For this review, take the finished solid that the model builds, in its own axes (mm). Face numbers are marked on the shaded views. Coordinates: 2 decimals unless noted, no trailing zeros. Loops run counter-clockwise (first coordinate to the right, second up) from the corner with the lowest first, then second, coordinate; pieces in that order, holes last. Notation, with made-up numbers: (27.5, 10) - (39.5, 10) arc R15 ccw to (39.5, 34) - close; hole circle Ø3 at (69, 39). An arc over 180 degrees is marked (long way). Answer as a JSON object with one key per item and string values. Group by question number.
Item 1: We need section B-B (x = 0). State how many separate pieces and enclosed holes the cut face has, then the cut area to 3 significant figures.
Item 2: We need section A-A (y = -5.5). Give the boundary of the cut face in (x, z), then the cut area to 3 significant figures.
Item 3: To check wall thickness, follow line 1 (Z direction, x = 0, y = -4.25); line 2 (Z direction, x = -16, y = -7.25); line 3 (X direction, y = -9, z = 7.5). State the ranges of each line that lie inside material, in increasing order.
Item 4: Mouldability with a two-part tool opening along X and no side actions: class the marked faces 1, 2, 3 and 4 as released by +X, released by -X, zero draft, split by the parting line, or undercut.
Item 5: Clearance check with flat-ended pins moving along their axes: pin 1 (3 mm diameter, centred on x = 2, z = 15.5, fed in from -Y); pin 2 (8 mm diameter, centred on x = 15, z = -2, fed in from -Y). State where each tip first meets the part, or that it passes through.
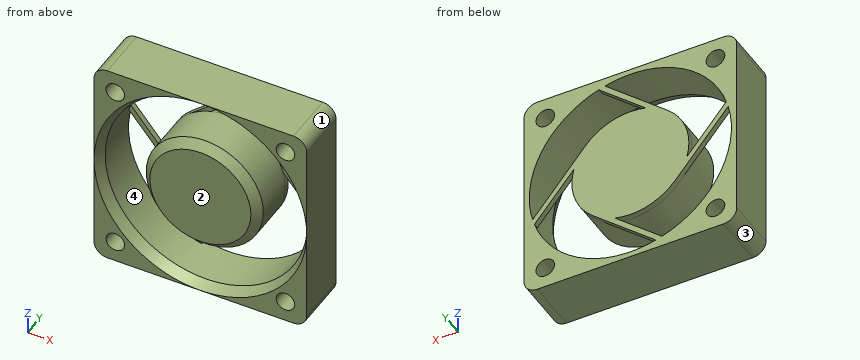
from build123d import *

# Parameters (mm, degrees)
F0_R     = 1.75
F0_R_2   = 19
F1_DEPTH = 10
F3_DEPTH = 1
F4_R     = 11
F5_DEPTH = 9
F7_SIZE2 = 0.99999
F7_SIZE  = 1.99999


# Not quite as in the source:
# - a fillet or chamfer that OpenCascade refuses, or shapes differently, is made with other operations: its cross-section is extruded or revolved along the edge and cut away or added
# - a fillet or chamfer is up to 0.001 mm smaller than in the source, because OpenCascade refuses the exact size


with BuildPart() as f1:
    # F0 (on Front) → F1 (new body)
    with BuildSketch(Plane.XZ):
        with BuildLine():
            Line((-17.5, -20), (17.5, -20))
            ThreePointArc((17.5, -20), (19.267766953, -19.267766953), (20, -17.5))
            Line((20, -17.5), (20, 17.5))
            ThreePointArc((20, 17.5), (19.267766953, 19.267766953), (17.5, 20))
            Line((17.5, 20), (-17.5, 20))
            ThreePointArc((-17.5, 20), (-19.267766953, 19.267766953), (-20, 17.5))
            Line((-20, 17.5), (-20, -17.5))
            ThreePointArc((-20, -17.5), (-19.267766953, -19.267766953), (-17.5, -20))
        make_face()
        with Locations((-16, -16)):
            Circle(F0_R, mode=Mode.SUBTRACT)
        with Locations((16, -16)):
            Circle(F0_R, mode=Mode.SUBTRACT)
        with Locations((-16, 16)):
            Circle(F0_R, mode=Mode.SUBTRACT)
        Circle(F0_R_2, mode=Mode.SUBTRACT)
        with Locations((16, 16)):
            Circle(F0_R, mode=Mode.SUBTRACT)
    extrude(amount=F1_DEPTH)

    # F2 (on Front) → F3 (join)
    with BuildSketch(Plane.XZ):
        with BuildLine():
            Line((5.6323262572, 19.0855630677), (-7.0706637066, 8.4264888743))
            ThreePointArc((-7.0706637066, 8.4264888743), (-10.5017983633, 3.2729544964), (-10.6060673084, -2.9174194506))
            Line((-10.6060673084, -2.9174194506), (-18.3195186246, 6.2751138669))
            Line((-18.3195186246, 6.2751138669), (-19.0855630677, 5.6323262572))
            Line((-19.0855630677, 5.6323262572), (-8.4264888743, -7.0706637066))
            ThreePointArc((-8.4264888743, -7.0706637066), (-3.2729544964, -10.5017983633), (2.9174194506, -10.6060673084))
            Line((2.9174194506, -10.6060673084), (-6.2751138669, -18.3195186246))
            Line((-6.2751138669, -18.3195186246), (-5.6323262572, -19.0855630677))
            Line((-5.6323262572, -19.0855630677), (7.0706637066, -8.4264888743))
            ThreePointArc((7.0706637066, -8.4264888743), (10.5017983633, -3.2729544964), (10.6060673084, 2.9174194506))
            Line((10.6060673084, 2.9174194506), (18.3195186246, -6.2751138669))
            Line((18.3195186246, -6.2751138669), (19.0855630677, -5.6323262572))
            Line((19.0855630677, -5.6323262572), (8.4264888743, 7.0706637066))
            ThreePointArc((8.4264888743, 7.0706637066), (3.2729544964, 10.5017983633), (-2.9174194506, 10.6060673084))
            Line((-2.9174194506, 10.6060673084), (6.2751138669, 18.3195186246))
            Line((6.2751138669, 18.3195186246), (5.6323262572, 19.0855630677))
        make_face()
    extrude(amount=F3_DEPTH)

    # F4 (on face) → F5 (join)
    with BuildSketch(Plane.XZ.offset(1)):
        Circle(F4_R)
    extrude(amount=F5_DEPTH)

    # F6: chamfer of 1.5 on 1 edges, made by hand

    # F6_s1 → F6_t2 (revolve, cut)
    with BuildSketch(Plane.XY):
        Polygon((11, -8.5), (9.5, -10), (11, -10), align=None)
    revolve(axis=Axis((0, -10, 0), (0, -1, 0)), mode=Mode.SUBTRACT)

    # F7 (size 2 and 1 in the source; OpenCascade refuses exactly that, so slightly less here)
    f7_edges = [f1.edges().sort_by_distance(p)[0] for p in [
        (-19, -10, 0),
    ]]
    f7_side = f1.faces().sort_by_distance((-19, -5, 0))[0]
    chamfer(f7_edges, length=F7_SIZE, length2=F7_SIZE2, reference=f7_side)


solid = f1.part
Check sheet entries:
{
 "1": {"separate pieces": "5", "enclosed holes": "0", "area": "238 mm2"},
 "2": {"outline": "(-20, -17.5) arc R2.5 ccw to (-17.5, -20) - (17.5, -20) arc R2.5 ccw to (20, -17.5) - (20, 17.5) arc R2.5 ccw to (17.5, 20) - (-17.5, 20) arc R2.5 ccw to (-20, 17.5) - close; circle Ø22 at (0, 0); hole circle Ø38 at (0, 0); hole circle Ø3.5 at (-16, -16); hole circle Ø3.5 at (-16, 16); hole circle Ø3.5 at (16, -16); hole circle Ø3.5 at (16, 16)", "area": "802 mm2"},
 "3": {"line 1": "z = -20 to -19, -11 to 11, 19 to 20", "line 2": "z = -20 to -17.75, -14.25 to -10.25, 10.25 to 14.25, 17.75 to 20", "line 3": "x = -20 to -18, -7.35 to 7.35, 18 to 20"},
 "4": {"face 1": "released by +X", "face 2": "zero draft", "face 3": "released by -X", "face 4": "undercut"},
 "5": {"pin 1": "stops at y = -1", "pin 2": "stops at y = -8.27"}
}
